```python
from build123d import *

# Parameters (mm, degrees)
SKETCH1_R           = 1.1
BOSS_EXTRUDE1_DEPTH = 4.4
BOSS_EXTRUDE2_DEPTH = 2.9
SKETCH3_R           = 2
CUT_EXTRUDE1_DEPTH  = 2.5
BOSS_EXTRUDE3_DEPTH = 1.6
SKETCH6_R           = 3.25
CUT_EXTRUDE2_DEPTH  = 10.869724242


with BuildPart() as part:
    # Sketch1 → Boss-Extrude1 (new body)
    with BuildSketch(Plane(origin=(0, 0, 0), x_dir=(1, 0, 0), z_dir=(0, 1, 0))):
        with BuildLine():
            Line((-3.1, -37.371647007), (-3.1, -34.998978499))
            ThreePointArc((-3.1, -34.998978499), (-7.096909, -34.411805803), (-11, -33.369724242))
            Line((-11, -33.369724242), (-11, -27.630275758))
            Line((-11, -27.630275758), (11, -27.630275758))
            Line((11, -27.630275758), (11, -33.369724242))
            ThreePointArc((11, -33.369724242), (7.096909, -34.411805803), (3.1, -34.998978499))
            Line((3.1, -34.998978499), (3.1, -37.371647007))
            ThreePointArc((3.1, -37.371647007), (0, -37.5), (-3.1, -37.371647007))
        make_face()
        with Locations((-8, -30.5)):
            Circle(SKETCH1_R, mode=Mode.SUBTRACT)
        with Locations((8, -30.5)):
            Circle(SKETCH1_R, mode=Mode.SUBTRACT)
    extrude(amount=BOSS_EXTRUDE1_DEPTH)

    # Sketch2 → Boss-Extrude2 (add)
    with BuildSketch(Plane(origin=(0, 4.4, 0), x_dir=(1, 0, 0), z_dir=(0, 1, 0))):
        with BuildLine():
            Line((3.1, -37.371647007), (3.1, -35.665529577))
            ThreePointArc((3.1, -35.665529577), (0, -35.8), (-3.1, -35.665529577))
            Line((-3.1, -35.665529577), (-3.1, -37.371647007))
            ThreePointArc((-3.1, -37.371647007), (0, -37.5), (3.1, -37.371647007))
        make_face()
    extrude(amount=BOSS_EXTRUDE2_DEPTH)

    # Sketch3 → Cut-Extrude1 (cut)
    with BuildSketch(Plane(origin=(0, 4.4, 0), x_dir=(1, 0, 0), z_dir=(0, 1, 0))):
        with Locations((-8, -30.5)):
            Circle(SKETCH3_R)
        with Locations((8, -30.5)):
            Circle(SKETCH3_R)
    extrude(amount=-CUT_EXTRUDE1_DEPTH, mode=Mode.SUBTRACT)

    # Sketch5 → Boss-Extrude3 (add)
    with BuildSketch(Plane.XZ):
        with BuildLine():
            Line((-4.85, 34.799655113), (-4.85, 27.630275758))
            Line((-4.85, 27.630275758), (4.85, 27.630275758))
            Line((4.85, 27.630275758), (4.85, 34.799655113))
            ThreePointArc((4.85, 34.799655113), (3.976249169, 34.910284137), (3.1, 34.998978499))
            Line((3.1, 34.998978499), (3.1, 37.371647007))
            ThreePointArc((3.1, 37.371647007), (0, 37.5), (-3.1, 37.371647007))
            Line((-3.1, 37.371647007), (-3.1, 34.998978499))
            ThreePointArc((-3.1, 34.998978499), (-3.976249169, 34.910284137), (-4.85, 34.799655113))
        make_face()
    extrude(amount=BOSS_EXTRUDE3_DEPTH)

    # Sketch6 → Cut-Extrude2 (cut, through all)
    with BuildSketch(Plane(origin=(0, 0, 27.630275758), x_dir=(-1, 0, 0), z_dir=(0, 0, -1))):
        with Locations((0, -1.35)):
            Circle(SKETCH6_R)
    extrude(amount=-CUT_EXTRUDE2_DEPTH, mode=Mode.SUBTRACT)


solid = part.part
```
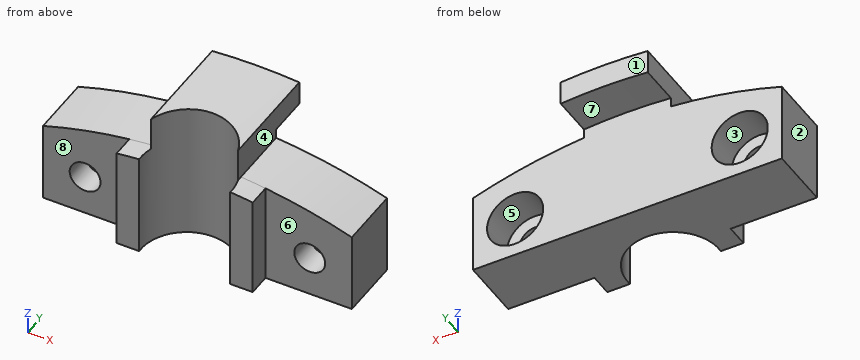
Could you check a few things on this model? Use its own coordinates, in mm. Face numbers are marked on the shaded views. A direction names the side the tool comes from. Round coordinates to 2 decimals unless told otherwise and drop trailing zeros. Loops run counter-clockwise (first coordinate to the right, second up) from the corner with the lowest first, then second, coordinate; pieces in that order, holes last. Notation, with made-up numbers: (12, 78) - (56, 78) arc R19 ccw to (56, 107) - close; hole circle Ø1 at (-27, 26). An arc over 180 degrees is marked (long way). Use CSV: the item, a comma, the result in double quotes.
Item 1: If we section it at C-C on z = 33: List the corners of the cut face in (x, y) for me.
Here are the results:
outline,"(-11, 0) - (-4.85, 0) - (-4.85, -1.6) - (-3.24, -1.6) arc R3.25 cw (long way) to (3.24, -1.6) - (4.85, -1.6) - (4.85, 0) - (11, 0) - (11, 4.4) - (-11, 4.4) - close"
Item 2: If we section it at D-D on y = 1: List the corners of the cut face in (x, z) for me (3 decimals), then the cut area to 3 significant figures.
Here are the results:
outline,"(-11, 27.63) - (-2.245, 27.63) - (-2.245, 37.433) arc R37.5 ccw to (-3.1, 37.372) - (-3.1, 34.999) arc R35.136 ccw to (-11, 33.37) - close; (2.245, 27.63) - (11, 27.63) - (11, 33.37) arc R35.136 ccw to (3.1, 34.999) - (3.1, 37.372) arc R37.5 ccw to (2.245, 37.433) - close; hole circle Ø2.2 at (-8, 30.5); hole circle Ø2.2 at (8, 30.5)"
area,"115 mm²"
Item 3: For the marked faces 4, 5, 6, 7 and 8, which set-ups out of +Z, -Z, +X, -X, +Y, -Y let a thin tool reach every point of the face, with its end or its side?
Here are the results:
face 4,"+Z, +X, +Y, -Y"
face 5,"+Y"
face 6,"+Z, -Z, +X, -Y"
face 7,"-Z, +Y"
face 8,"+Z, -Z, -X, -Y"
Item 4: I need wall thicknesses on L1, parallel to X at y = 3.2, z = 30.5; L2, parallel to Y at x = -7.25, z = 31.75; L3, parallel to X at y = 3.5, z = 35.25. Which ranges of each line are inside material? Lowest first, please. Write a range as [from, to].
Here are the results:
L1,"x = [-11, -10], [-6, 6], [10, 11]"
L2,"y = [0, 1.9]"
L3,"x = [-3.1, 3.1]"
Item 5: If we section it at A-A on x = -8: List the corners of the cut face in (y, z) for me.
Here are the results:
outline,"(0, 27.63) - (4.4, 27.63) - (4.4, 28.5) - (1.9, 28.5) - (1.9, 29.4) - (0, 29.4) - close; (0, 31.6) - (1.9, 31.6) - (1.9, 32.5) - (4.4, 32.5) - (4.4, 34.21) - (0, 34.21) - close"
Item 6: If we section it at B-B on y = -0.75: List the corners of the cut face in (x, z) for me, then the cut area to 3 significant figures.
Here are the results:
outline,"(-4.85, 27.63) - (-3.19, 27.63) - (-3.19, 34.99) arc R35.14 ccw to (-4.85, 34.8) - close; (3.19, 27.63) - (4.85, 27.63) - (4.85, 34.8) arc R35.14 ccw to (3.19, 34.99) - close"
area,"24.1 mm²"
Item 7: If we mould it in two halves opening along X, with no side actions, what happens to the marked faces 1, 2 and 3? For each: pulls with the +X half, pulls with the -X half, needs draft (parallel to the pull), parting line crosses it, or undercut.
Here are the results:
face 1,"needs draft"
face 2,"pulls with the -X half"
face 3,"undercut"
Item 8: Will these pins go through, and if not, where does the flat tip stop? pin 1 (5 mm diameter, centred on x = 9.5, z = 32, fed in from -Y); pin 2 (4 mm diameter, centred on x = 7.5, z = 30.5, fed in from +Y); pin 3 (3 mm diameter, centred on x = -3.5, y = 6, fed in from +Z).
Here are the results:
pin 1,"stops at y = 0"
pin 2,"stops at y = 4.4"
pin 3,"stops at z = 37.45"
